Could you check a few things on this model? Use its own coordinates, in mm. Give positions to 0.01 mm unless a question says otherwise; leave off trailing zeros. Order: outer loops, then holes, each group sorted by start corner. A loop starts at its lowest first (then second) coordinate and runs counter-clockwise, first axis right, second up. Notation, with made-up numbers: (-37, 49.5) -> (19, 49.5) arc R14 cw to (19, 55.5) -> close; hole circle Ø3 at (33, 53.5). An arc over 180 degrees is marked (long way). Answer as CSV lines item,"result". Start each with the question number.
(1) I need wall thicknesses on L1, parallel to X at y = 15, z = 2.15. Which ranges of the line are inside material? Lowest first, please.
(2) I want a section at B-B (z = 1.3). Please give me the cut outline in (x, y).
(3) I want a section at D-D (y = 15.5). Please give me the cut outline in (x, z), plus the area to 3 significant figures.
(4) Will these pins go through, and if not, where does the flat tip stop? pin 1 Ø0.6 at (x, z) = (-5, 1) entering from +Y; pin 2 Ø1.5 at (x, z) = (37.5, 2.5) entering from -Y; pin 3 Ø1.6 at (x, z) = (-4, 1) entering from -Y; pin 4 Ø0.5 at (x, z) = (33.5, 2.5) entering from -Y.
(5) I want a section at C-C (x = 29.5). Please give me the cut outline in (y, z), plus the area to 3 significant figures.
(6) I want a section at A-A (y = 54). Please give me the cut outline in (x, z).
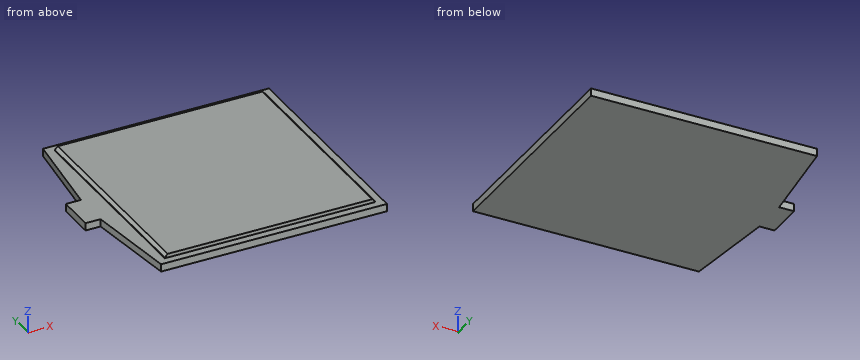
```python
from build123d import *

# Parameters (mm, degrees)
PAD_DEPTH        = 2
SKETCH001_W      = 55.9
SKETCH001_H      = 55.9
PAD001_DEPTH     = 1
CHAMFER_SIZE2    = 0.8
CHAMFER_SIZE     = 0.8
CHAMFER001_SIZE2 = 0.8
CHAMFER001_SIZE  = 0.8


with BuildPart() as part:
    # Sketch → Pad (new body)
    with BuildSketch(Plane.XY):
        Polygon((0, 60), (60, 60), (60, 0), (0, 0), (-3, 25), (-7, 25), (-7, 35), (-3, 35), align=None)
    extrude(amount=PAD_DEPTH)

    # Sketch001 → Pad001 (join)
    with BuildSketch(Plane.XY.offset(2)):
        with Locations((30, 30)):
            Rectangle(SKETCH001_W, SKETCH001_H)
    extrude(amount=PAD001_DEPTH)

    # Chamfer
    chamfer_edges = [part.edges().sort_by_distance(p)[0] for p in [
        (2.05, 30, 3),
    ]]
    chamfer_side = part.faces().sort_by_distance((2.05, 30, 2.5))[0]
    chamfer(chamfer_edges, length=CHAMFER_SIZE, length2=CHAMFER_SIZE2, reference=chamfer_side)

    # Chamfer001
    chamfer001_edges = [part.edges().sort_by_distance(p)[0] for p in [
        (57.95, 30, 3),
    ]]
    chamfer001_side = part.faces().sort_by_distance((30.4, 30, 3))[0]
    chamfer(chamfer001_edges, length=CHAMFER001_SIZE, length2=CHAMFER001_SIZE2, reference=chamfer001_side)


solid = part.part
```
Final values:
1,L1,"2.05 to 57.95"
2,outline,"(-7, 25) -> (-3, 25) -> (0, 0) -> (60, 0) -> (60, 60) -> (0, 60) -> (-3, 35) -> (-7, 35) -> close"
3,outline,"(-1.86, 0) -> (60, 0) -> (60, 2) -> (57.95, 2) -> (57.95, 2.2) -> (57.15, 3) -> (2.85, 3) -> (2.05, 2.2) -> (2.05, 2) -> (-1.86, 2) -> close"
3,area,"179 mm²"
4,pin 1,"y = 35"
4,pin 2,"y = 0"
4,pin 3,"y = 25"
4,pin 4,"y = 2.05"
5,outline,"(0, 0) -> (60, 0) -> (60, 2) -> (57.95, 2) -> (57.95, 3) -> (2.05, 3) -> (2.05, 2) -> (0, 2) -> close"
5,area,"176 mm²"
6,outline,"(-0.72, 0) -> (60, 0) -> (60, 2) -> (57.95, 2) -> (57.95, 2.2) -> (57.15, 3) -> (2.85, 3) -> (2.05, 2.2) -> (2.05, 2) -> (-0.72, 2) -> close"
